Could you check a few things on this model? Use its own coordinates, in mm. Face numbers are marked on the shaded views. A direction names the side the tool comes from. Coordinates: 2 decimals unless noted, no trailing zeros. Write each loop counter-clockwise with the first axis right and the second up, starting at its lowest first coordinate (ties: lowest second). Pieces come first, ordered by that corner, then holes. Notation, with made-up numbers: M 4.25,4 L 13.25,4 A27 cw 13.25,27 Z; hole C 37.25,23.5 d8. An arc over 180 degrees is marked long. Write item = value, one per line.
```python
from build123d import *

# Parameters (mm, degrees)
ESQUISSE1_W        = 90
ESQUISSE1_H        = 90
BOSS_EXTRU_1_DEPTH = 20
ESQUISSE2_R        = 6
BOSS_EXTRU_2_DEPTH = 277
ESQUISSE3_W        = 80
ESQUISSE3_H        = 80
BOSS_EXTRU_3_DEPTH = 2.9
ESQUISSE4_W        = 80
ESQUISSE4_H        = 80
BOSS_EXTRU_4_DEPTH = 0.1


with BuildPart() as part:
    # Esquisse1 → Boss.-Extru.1 (new body)
    with BuildSketch(Plane(origin=(0, 0, 0), x_dir=(0, 0, -1), z_dir=(1, 0, 0))):
        with Locations((30.929303344, -12.964038863)):
            Rectangle(ESQUISSE1_W, ESQUISSE1_H)
    extrude(amount=BOSS_EXTRU_1_DEPTH)

    # Esquisse2 → Boss.-Extru.2 (add)
    with BuildSketch(Plane(origin=(0, 32.035961137, 0), x_dir=(1, 0, 0), z_dir=(0, 1, 0))):
        with Locations(Location((10, 30.929303344, 0), (0, 0, 90))):
            Circle(ESQUISSE2_R)
    extrude(amount=BOSS_EXTRU_2_DEPTH)

    # Esquisse3 → Boss.-Extru.3 (add)
    with BuildSketch(Plane(origin=(0, 309.035961137, 0), x_dir=(1, 0, 0), z_dir=(0, 1, 0))):
        with Locations((-20, 30.929303344)):
            Rectangle(ESQUISSE3_W, ESQUISSE3_H)
    extrude(amount=BOSS_EXTRU_3_DEPTH)

    # Esquisse4 → Boss.-Extru.4 (add)
    with BuildSketch(Plane(origin=(0, 311.935961137, 0), x_dir=(1, 0, 0), z_dir=(0, 1, 0))):
        with Locations((-20, 30.929303344)):
            Rectangle(ESQUISSE4_W, ESQUISSE4_H)
    extrude(amount=BOSS_EXTRU_4_DEPTH)


solid = part.part
```
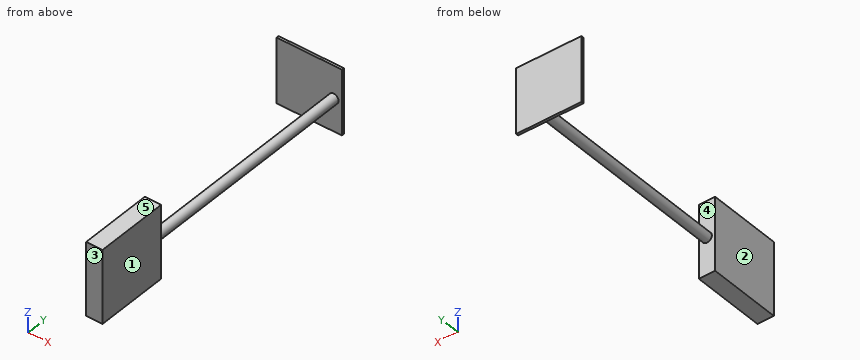
Item 1: Imagine slicing it at D-D (x = -23.5). Write out the boundary of the cut face in (y, z).
Numbers:
outline = M 309.04,-70.93 L 312.04,-70.93 L 312.04,9.07 L 309.04,9.07 Z
Item 2: If I drill on line 1 along Y through (x, z) = (10, -4.5); line 2 along Y through (x, z) = (-24, -55); line 3 along Y through (x, z) = (7, -71.5), over which ranges is the centre line in solid material (lowest first)?
Numbers:
line_1 = -57.96 to 32.04, 309.04 to 312.04
line_2 = 309.04 to 312.04
line_3 = -57.96 to 32.04
Item 3: For the marked faces 1 and 2, which set-ups out of +Z, -Z, +X, -X, +Y, -Y let a thin tool reach every point of the face, with its end or its side?
Numbers:
face_1 = +Z, -Z, +X, +Y, -Y
face_2 = +Z, -Z, -X, -Y
Item 4: If we mould it in two halves opening along Y, with no side actions, what happens to the marked faces 3, 4 and 5? For each: pulls with the +Y half, pulls with the -Y half, needs draft (parallel to the pull), parting line crosses it, or undercut.
Numbers:
face_3 = pulls with the -Y half
face_4 = undercut
face_5 = needs draft
Item 5: Imagine slicing it at C-C (y = 267). Write out the boundary of the cut face in (x, z).
Numbers:
outline = C 10,-30.93 d12
Item 6: Imagine slicing it at A-A (z = 4). Write out the boundary of the cut face in (x, y).
Numbers:
outline = M -60,309.04 L 20,309.04 L 20,312.04 L -60,312.04 Z; M 0,-57.96 L 20,-57.96 L 20,32.04 L 0,32.04 Z
Item 7: Imagine slicing it at B-B (x = 10). Write out the boundary of the cut face in (y, z).
Numbers:
outline = M -57.96,-75.93 L 32.04,-75.93 L 32.04,-36.93 L 309.04,-36.93 L 309.04,-70.93 L 312.04,-70.93 L 312.04,9.07 L 309.04,9.07 L 309.04,-24.93 L 32.04,-24.93 L 32.04,14.07 L -57.96,14.07 Z
Item 8: I'm going to push flat-ended pins straight in: P1, Ø3.5, axis at x = -38, y = 310.5, coming from the -Z side; P2, Ø2, axis at x = 4, y = 51, coming from the -Z side; P3, Ø2.5, axis at x = -31.5, y = 311.5, coming from the +Z side. Where does each tip first touch, or does it pass through?
Numbers:
P1 = -70.93
P2 = -34.25
P3 = 9.07
